from build123d import *

# Parameters (mm, degrees)
SKETCH1_R           = 6.5
BOSS_EXTRUDE1_DEPTH = 9
SKETCH3_R           = 4.5
CUT_EXTRUDE1_DEPTH  = 7
SKETCH2_R           = 2.5
CUT_EXTRUDE2_DEPTH  = 3
FILLET2_R           = 1


with BuildPart() as part:
    # Sketch1 → Boss-Extrude1 (new body)
    with BuildSketch(Plane(origin=(0, 0, 0), x_dir=(1, 0, 0), z_dir=(0, 1, 0))):
        Circle(SKETCH1_R)
    extrude(amount=BOSS_EXTRUDE1_DEPTH)

    # Sketch3 → Cut-Extrude1 (cut)
    with BuildSketch(Plane.XZ):
        Circle(SKETCH3_R)
    extrude(amount=-CUT_EXTRUDE1_DEPTH, mode=Mode.SUBTRACT)

    # Sketch2 → Cut-Extrude2 (cut)
    with BuildSketch(Plane(origin=(0, 9, 0), x_dir=(1, 0, 0), z_dir=(0, 1, 0))):
        Circle(SKETCH2_R)
    extrude(amount=-CUT_EXTRUDE2_DEPTH, mode=Mode.SUBTRACT)

    # Fillet2
    fillet2_edges = [part.edges().sort_by_distance(p)[0] for p in [
        (-2.5, 7, 0),
    ]]
    fillet(fillet2_edges, radius=FILLET2_R)


solid = part.part
Source: CAD feature listing. Evaluate the final solid. Frame: model axes, mm. Coordinates: 2 decimals unless noted, no trailing zeros. Loops run counter-clockwise (first coordinate to the right, second up) from the corner with the lowest first, then second, coordinate; pieces in that order, holes last. Notation, with made-up numbers: (44.25, -15) -> (77.25, -15) arc R17 ccw to (77.25, 5) -> close; hole circle Ø11 at (28.25, 83.5). An arc over 180 degrees is marked (long way). Answer in a Markdown table with one row per item. Add a question column.
Q1. Section D-D on z = 5.75. Return the cut outline in (x, y), and give its area (3 significant figures).
Q2. Section B-B on x = 0. Return the cut outline in (y, z), and give its area (3 significant figures).
Q3. Ray query, line 1 along X through (y, z) = (8.25, 0); line 2 along Z through (x, y) = (0, 3.5). Return the intervals inside material, ascending.
Q4. Pull-direction query (Z, two-part tool) for faces 1 (the face through (0, 7, -4)), 2 (the face through (-4.42, 0, -1.54)), 3 (the face through (-0.59, 3.45, 4.46)), 4 (the face through (-5.158, 4.437, 3.955)); classes: pulls with the +Z half, pulls with the -Z half, needs draft (parallel to the pull), parting line crosses it, or undercut.
Q5. Section A-A on z = 0. Return the cut outline in (x, y), and give its area (3 significant figures).
Q6. Section C-C on y = 6. Return the cut outline in (x, z).
Q7. Contact query for flat-ended pins moving along their axis: pin 1 Ø3 at (y, z) = (3, -2) entering from +X; pin 2 Ø5 at (y, z) = (3.5, -3) entering from -X; pin 3 Ø4 at (x, z) = (0, 0) entering from -Y; pin 4 Ø5.5 at (x, z) = (0, 0) entering from -Y. Output: stop coordinate, or through.
Computed values:
| question | item | result |
|---|---|---|
| 1 | outline | (-3.03, 0) -> (3.03, 0) -> (3.03, 9) -> (-3.03, 9) -> close |
| 1 | area | 54.6 mm^2 |
| 2 | outline | (0, -6.5) -> (9, -6.5) -> (9, -2.5) -> (8, -2.5) arc R1 ccw to (7, -3.5) -> (7, -4.5) -> (0, -4.5) -> close; (0, 4.5) -> (7, 4.5) -> (7, 3.5) arc R1 ccw to (8, 2.5) -> (9, 2.5) -> (9, 6.5) -> (0, 6.5) -> close |
| 2 | area | 43.6 mm^2 |
| 3 | line 1 | x = -6.5 to -2.5, 2.5 to 6.5 |
| 3 | line 2 | z = -6.5 to -4.5, 4.5 to 6.5 |
| 4 | face 1 | undercut |
| 4 | face 2 | needs draft |
| 4 | face 3 | undercut |
| 4 | face 4 | parting line crosses it |
| 5 | outline | (-6.5, 0) -> (-4.5, 0) -> (-4.5, 7) -> (-3.5, 7) arc R1 ccw to (-2.5, 8) -> (-2.5, 9) -> (-6.5, 9) -> close; (2.5, 8) arc R1 ccw to (3.5, 7) -> (4.5, 7) -> (4.5, 0) -> (6.5, 0) -> (6.5, 9) -> (2.5, 9) -> close |
| 5 | area | 43.6 mm^2 |
| 6 | outline | circle Ø13 at (0, 0); hole circle Ø9 at (0, 0) |
| 7 | pin 1 | stops at x = 6.48 |
| 7 | pin 2 | stops at x = -6.48 |
| 7 | pin 3 | passes through |
| 7 | pin 4 | stops at y = 7.34 |
